Build history of the part. All positions in model axes, mm. A direction names the side the tool comes from. Coordinates: 2 decimals unless noted, no trailing zeros. Loops run counter-clockwise (first coordinate to the right, second up) from the corner with the lowest first, then second, coordinate; pieces in that order, holes last. Notation, with made-up numbers: (28, 31.5) - (65, 31.5) arc R21 ccw to (65, 62.5) - close; hole circle Ø11 at (52.5, -25). An arc over 180 degrees is marked (long way). One line per item, written item: value.
```python
from build123d import *

# Parameters (mm, degrees)
EXTRUDE_1_DEPTH = 4.8
EXTRUDE_2_DEPTH = 4.8


# Read off the part's stored shape, not the designer's step: 交差1
with BuildPart() as part:
    # ｽｹｯﾁ1 → 押し出し-薄板1 (new body)
    with BuildSketch(Plane.XY):
        with BuildLine():
            Line((-22.5, 14.23), (22.5, 14.23))
            ThreePointArc((22.5, 14.23), (36.73, 0), (22.5, -14.23))
            Line((22.5, -14.23), (-22.5, -14.23))
            ThreePointArc((-22.5, -14.23), (-36.73, 0), (-22.5, 14.23))
        make_face()
        with BuildLine():
            Line((-22.5, 13.42), (22.5, 13.42))
            ThreePointArc((22.5, 13.42), (35.92, 0), (22.5, -13.42))
            Line((22.5, -13.42), (-22.5, -13.42))
            ThreePointArc((-22.5, -13.42), (-35.92, 0), (-22.5, 13.42))
        make_face(mode=Mode.SUBTRACT)
    extrude(amount=EXTRUDE_1_DEPTH)


with BuildPart() as body_2:
    # ｽｹｯﾁ2 → 押し出し-薄板2 (new body)
    with BuildSketch(Plane.XY.offset(4.8)):
        with BuildLine():
            Line((-22.5, -14.23), (22.5, -14.23))
            ThreePointArc((22.5, -14.23), (36.73, 0), (22.5, 14.23))
            Line((22.5, 14.23), (-22.5, 14.23))
            ThreePointArc((-22.5, 14.23), (-36.73, 0), (-22.5, -14.23))
        make_face()
        with BuildLine():
            Line((-22.5, -13.93), (22.5, -13.93))
            ThreePointArc((22.5, -13.93), (36.43, 0), (22.5, 13.93))
            Line((22.5, 13.93), (-22.5, 13.93))
            ThreePointArc((-22.5, 13.93), (-36.43, 0), (-22.5, -13.93))
        make_face(mode=Mode.SUBTRACT)
    extrude(amount=-EXTRUDE_2_DEPTH)


solid = part.part
```
Item 1: Cut at C-C, the plane z = 3.3. Write the cut outline in (x, y), then the cut area to 3 significant figures.
Check result:
outline: (-22.5, -14.23) - (22.5, -14.23) arc R14.23 ccw to (22.5, 14.23) - (-22.5, 14.23) arc R14.23 ccw to start; hole (-22.5, -13.42) - (22.5, -13.42) arc R13.42 ccw to (22.5, 13.42) - (-22.5, 13.42) arc R13.42 ccw to start
area: 143 mm^2
Item 2: Pull direction X, two halves, no side cores. Call faces 3 (the face through (-35.917, -0.295, 2.366)), 4 (the face through (0, -14.23, 2)), 5 (the face through (36.727, 0.313, 2.366)), 6 (the face through (0, -13.42, 2)): released by +X, released by -X, zero draft, split by the parting line, or undercut.
Check result:
face 3: undercut
face 4: zero draft
face 5: released by +X
face 6: undercut
Item 3: Tool access for faces 1 (the face through (35.917, 0.295, 2.366)), 2 (the face through (0, 14.23, 2)): list every direction of +Z, -Z, +X, -X, +Y, -Y with a clear straight run to the whole face (end or side of a thin tool).
Check result:
face 1: +Z, -Z
face 2: +Z, -Z, +X, -X, +Y
Item 4: Cut at B-B, the plane y = 0. Write the cut outline in (x, z), then the cut area to 3 significant figures.
Check result:
outline: (-36.73, 0) - (-35.92, 0) - (-35.92, 4.8) - (-36.73, 4.8) - close; (35.92, 0) - (36.73, 0) - (36.73, 4.8) - (35.92, 4.8) - close
area: 7.78 mm^2
Item 5: Cut at A-A, the plane x = -9. Write the cut outline in (y, z).
Check result:
outline: (-14.23, 0) - (-13.42, 0) - (-13.42, 4.8) - (-14.23, 4.8) - close; (13.42, 0) - (14.23, 0) - (14.23, 4.8) - (13.42, 4.8) - close
Item 6: Probe probe 1 along X at (y, z) = (-0.5, 3.65); probe 2 along Y at (x, z) = (-14, 0.6); probe 3 along X at (y, z) = (3.25, 1). List the from-to ranges inside material, lowest first. Write a range as from..to.
Check result:
probe 1: x = -36.72..-35.91, 35.91..36.72
probe 2: y = -14.23..-13.42, 13.42..14.23
probe 3: x = -36.35..-35.52, 35.52..36.35
